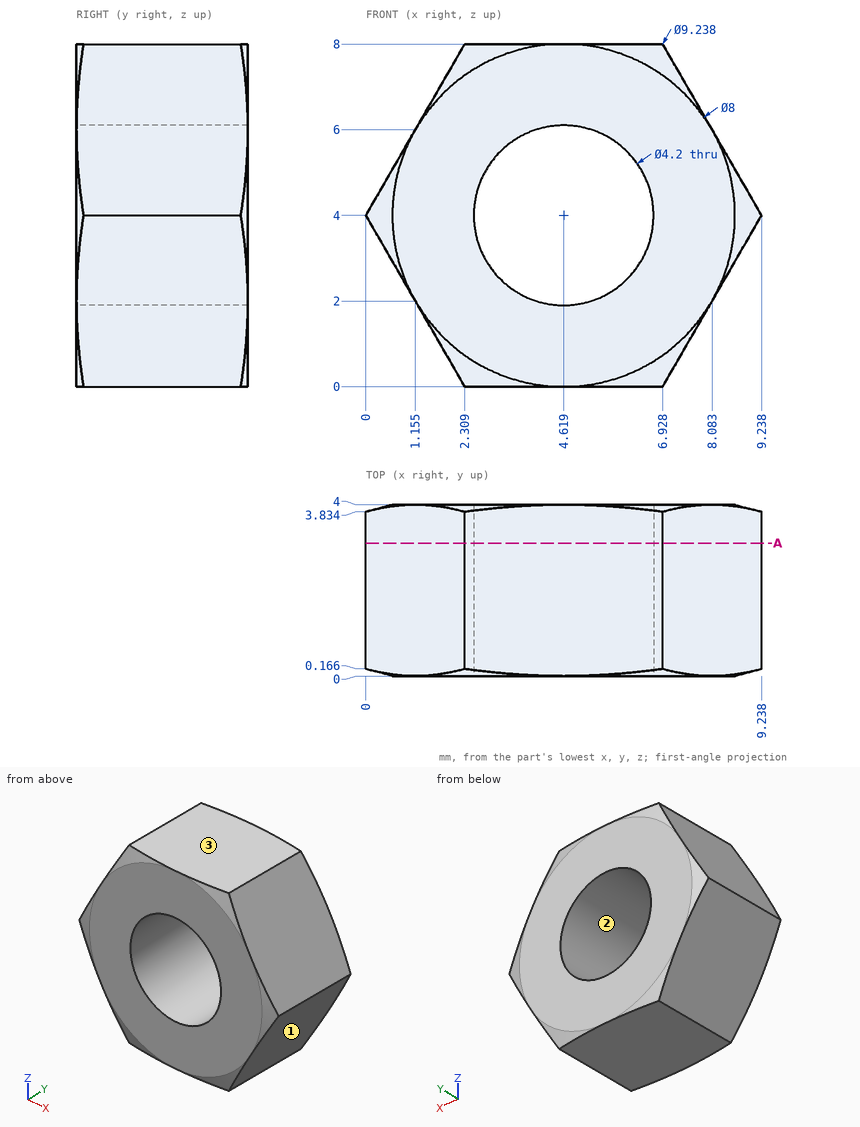
Input: dimensioned drawing with shaded views. Units: mm. Origin: part minimum x, y, z. Coordinates: 2 decimals unless noted, no trailing zeros. Loops run counter-clockwise (first coordinate to the right, second up) from the corner with the lowest first, then second, coordinate; pieces in that order, holes last. Notation, with made-up numbers: M 88,-33.5 L 115,-33.5 A8 cw 115,-28.5 Z; hole C 83.25,-12 d3. An arc over 180 degrees is marked long. One line per item, written item: value. Start each with the question number.
1) Pin query (flat end, axial travel): P1, Ø1, axis at x = 1, y = 3, coming from the -Z side; P2, Ø2, axis at x = 5, y = 2, coming from the -Z side. Return the tip coordinate at first contact, or that it passes through.
2) Material intervals for L1, parallel to Z at x = 4.75, y = 0.45 (1 decimal); L2, parallel to X at y = 2, z = 3.25 (1 decimal); L3, parallel to Z at x = 3.25, y = 0.35, sorted ascending. Write a range as from..to.
3) Draft query along Z for the marked faces 1, 2 and 3. Return one class per face: released by +Z, released by -Z, zero draft, split by the parting line, or undercut.
4) Cut plane A-A (y = 3.1). Return loops of the section in (x, z).
Evaluation:
1. P1: z = 1.4
1. P2: z = 0
2. L1: 0..1.9, 6.1..8
2. L2: 0.4..2.7, 6.6..8.8
2. L3: 0..2.41, 5.59..8
3. face 1: released by -Z
3. face 2: undercut
3. face 3: released by +Z
4. outline: M 0,4 L 2.31,0 L 6.93,0 L 9.24,4 L 6.93,8 L 2.31,8 Z; hole C 4.62,4 d4.2
